```python
from build123d import *

# Parameters (mm, degrees)
F0_W     = 82.296
F0_H     = 36.83
F0_R     = 1.143
F1_DEPTH = 7.112
F2_DEPTH = 8.382
F3_DEPTH = 4.572


with BuildPart() as f1:
    # F0 (on Top) → F1 (new body)
    with BuildSketch(Plane.XY):
        with Locations((-41.148, 18.415)):
            Rectangle(F0_W, F0_H)
        with Locations((-78.867, 3.429)):
            Circle(F0_R, mode=Mode.SUBTRACT)
        with Locations((-3.429, 3.429)):
            Circle(F0_R, mode=Mode.SUBTRACT)
        Polygon((-7.62, 7.874), (-7.62, 1.524), (-74.676, 1.524), (-74.676, 7.874), (-80.264, 7.874), (-80.264, 27.686), (-74.676, 27.686), (-74.676, 34.036), (-7.62, 34.036), (-7.62, 27.686), (-2.032, 27.686), (-2.032, 7.874), align=None, mode=Mode.SUBTRACT)
        with Locations((-78.867, 32.131)):
            Circle(F0_R, mode=Mode.SUBTRACT)
        with Locations((-3.429, 32.131)):
            Circle(F0_R, mode=Mode.SUBTRACT)
    extrude(amount=F1_DEPTH)

    # F0 (on Top) → F2 (join)
    with BuildSketch(Plane.XY):
        Polygon((-74.676, 1.524), (-7.62, 1.524), (-7.62, 7.874), (-2.032, 7.874), (-2.032, 27.686), (-7.62, 27.686), (-7.62, 34.036), (-74.676, 34.036), (-74.676, 27.686), (-80.264, 27.686), (-80.264, 7.874), (-74.676, 7.874), align=None)
        Polygon((-8.89, 9.144), (-8.89, 2.794), (-73.406, 2.794), (-73.406, 9.144), (-78.994, 9.144), (-78.994, 26.416), (-73.406, 26.416), (-73.406, 32.766), (-8.89, 32.766), (-8.89, 26.416), (-3.302, 26.416), (-3.302, 9.144), align=None, mode=Mode.SUBTRACT)
    extrude(amount=F2_DEPTH)

    # F0 (on Top) → F3 (join)
    with BuildSketch(Plane.XY):
        Polygon((-73.406, 2.794), (-8.89, 2.794), (-8.89, 9.144), (-3.302, 9.144), (-3.302, 26.416), (-8.89, 26.416), (-8.89, 32.766), (-73.406, 32.766), (-73.406, 26.416), (-78.994, 26.416), (-78.994, 9.144), (-73.406, 9.144), align=None)
    extrude(amount=F3_DEPTH)


solid = f1.part
```
The model under review builds one solid part; all positions refer to its coordinate system, in mm. A direction names the side the tool comes from. Round coordinates to 2 decimals unless told otherwise and drop trailing zeros. Write each loop counter-clockwise with the first axis right and the second up, starting at its lowest first coordinate (ties: lowest second). Pieces come first, ordered by that corner, then holes. Notation, with made-up numbers: (31.25, 48) - (39.25, 48) arc R19 cw to (39.25, 83) - close; hole circle Ø7 at (25, 23). An arc over 180 degrees is marked (long way). Answer as CSV lines item,"result". Start each with the question number.
(1) We need section C-C on z = 5.75. State the section outline as (x, y) points, plus the area to 3 significant figures.
(2) For faces 4 (the cylindrical face through (-3.578, 33.264, 3.506)), 5 (the flat face through (-76, 26.416, 6)), list the 3-axis set-ups (+Z, -Z, +X, -X, +Y, -Y) from which the entire face can be reached by the end or side of a thin tool; tool diameter is ignored.
(3) We need section B-B on y = 19. State the section outline as (x, z) points.
(4) For pin 1 Ø0.6 at (x, z) = (-48, 7.5) entering from -Y; pin 2 Ø3 at (x, y) = (-25, 31) entering from +Z; pin 3 Ø1.8 at (x, y) = (-78.867, 3.429) entering from -Z; pin 4 Ø1.4 at (x, z) = (-51, 8) entering from +Y, all flat-tipped, find the tip position at first contact; note any pin that passes through.
(5) Draft analysis for pull direction Y (two halves, no side actions). For faces 1 (the flat face through (-42, 0, 4)), 2 (the flat face through (-3.302, 18, 6)), 3 (the flat face through (-41, 35, 7.112)), state which applies: pulls with the +Y half, pulls with the -Y half, needs draft (parallel to the pull), parting line crosses it, or undercut.
(6) To check wall thickness, follow line 1 (Y direction, x = -3.5, z = 1.25); line 2 (Y direction, x = -17, z = 6.5); line 3 (X direction, y = 22.5, z = 7.25). State the ranges of each line that lie inside material, in increasing order.
(7) We need section A-A on x = -49. State the section outline as (y, z) points.
Worked answers:
1,outline,"(-82.3, 0) - (0, 0) - (0, 36.83) - (-82.3, 36.83) - close; hole circle Ø2.29 at (-78.87, 3.43); hole circle Ø2.29 at (-78.87, 32.13); hole (-78.99, 9.14) - (-73.41, 9.14) - (-73.41, 2.79) - (-8.89, 2.79) - (-8.89, 9.14) - (-3.3, 9.14) - (-3.3, 26.42) - (-8.89, 26.42) - (-8.89, 32.77) - (-73.41, 32.77) - (-73.41, 26.42) - (-78.99, 26.42) - close; hole circle Ø2.29 at (-3.43, 3.43); hole circle Ø2.29 at (-3.43, 32.13)"
1,area,"888 mm²"
2,face 4,"+Z, -Z"
2,face 5,"+Z"
3,outline,"(-82.3, 0) - (0, 0) - (0, 7.11) - (-2.03, 7.11) - (-2.03, 8.38) - (-3.3, 8.38) - (-3.3, 4.57) - (-78.99, 4.57) - (-78.99, 8.38) - (-80.26, 8.38) - (-80.26, 7.11) - (-82.3, 7.11) - close"
4,pin 1,"y = 1.52"
4,pin 2,"z = 4.57"
4,pin 3,"through"
4,pin 4,"y = 34.04"
5,face 1,"pulls with the -Y half"
5,face 2,"undercut"
5,face 3,"needs draft"
6,line 1,"0 to 2.29, 4.57 to 30.99, 33.27 to 36.83"
6,line 2,"0 to 2.79, 32.77 to 36.83"
6,line 3,"-80.26 to -78.99, -3.3 to -2.03"
7,outline,"(0, 0) - (36.83, 0) - (36.83, 7.11) - (34.04, 7.11) - (34.04, 8.38) - (32.77, 8.38) - (32.77, 4.57) - (2.79, 4.57) - (2.79, 8.38) - (1.52, 8.38) - (1.52, 7.11) - (0, 7.11) - close"
